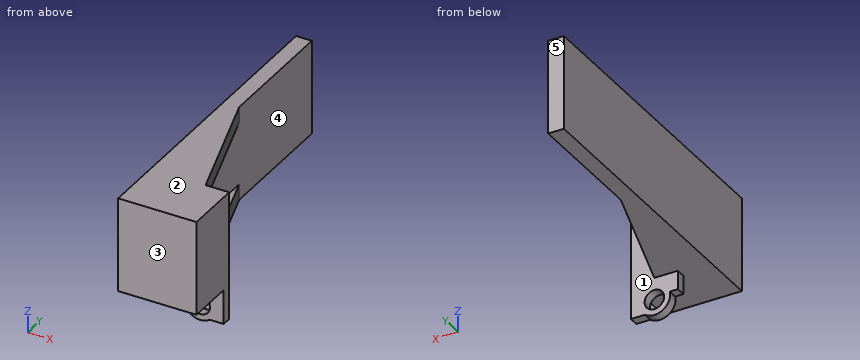
Autodesk Inventor part; units mm, degrees
ref_plane "YZ Plane" through (0, 0, 0) normal (1, 0, 0) x (0, 1, 0)
ref_plane "XZ Plane" through (0, 0, 0) normal (0, 1, 0) x (-1, 0, 0)
ref_plane "XY Plane" through (0, 0, 0) normal (0, 0, 1) x (1, 0, 0)
sketch "스케치2" plane through (0, 0, 0) normal (0, 1, 0) x (-1, 0, 0)
  circle A0 centre (0, 0) radius 3.1
  line L0 (0, 0) -> (0, 7)
  line L1 (0, 7) -> (7.475, 7)
  line L2 (7.475, 7) -> (7.475, 1.05)
  circle A1 centre (0, 0) radius 5
  line L3 (7.475, 1.05) -> (4.8885, 1.05)
  line L4 (0, 7) -> (-7.475, 7)
  line L5 (-7.475, 7) -> (-7.475, -5)
  line L6 (-7.475, -5) -> (0, -5)
  line L7 (-7.475, -5) -> (-7.475, -4)
  line L8 (-7.475, -4) -> (-3, -4)
  dimension "d0" = 6.2
  dimension "d1" = 7
  dimension "d2" = 7.475
  dimension "d3" = 5.95
  dimension "d4" = 10
  dimension "d5" = 7.475
  dimension "d21" = 1
extrude "돌출1" add sketch "스케치2" along normal blind 3 contours A1 | A1 L8 L5 L4 L0 | L0 L1 L2 L3 A1
sketch "스케치3" plane through (0, 3, 0) normal (0, 1, 0) x (1, 0, 0)
  line L0 (-7.475, -7) -> (7.475, -7)
  line L1 (-7.475, -7) -> (7.475, -7)
  line L2 (7.475, -7) -> (7.475, -37)
  line L3 (7.475, -37) -> (-7.475, -37)
  line L4 (-7.475, -37) -> (-7.475, -7)
  point P0 (0, 0)
  dimension "d8" = 30
extrude "돌출2" add sketch "스케치3" against normal blind 18
sketch "스케치11" plane through (0, 3, 0) normal (0, 1, 0) x (1, 0, 0)
  line L0 (-7.475, -37) -> (7.475, -37)
  line L1 (0, -37) -> (-17.4, -37)
  line L2 (-17.4, -37) -> (-17.4, -1.05)
  line L3 (-17.4, -1.05) -> (0, -1.05)
  line L4 (0, -1.05) -> (0, -37)
  line L5 (-7.475, -7) -> (7.475, -7)
  line L6 (-17.4, -37) -> (0, -37)
  line L7 (0, -37) -> (0, -7)
  line L8 (0, -7) -> (-17.4, -7)
  line L9 (-17.4, -7) -> (-17.4, -37)
  point P0 (0, 0)
  dimension "d40" = 17.4
extrude "돌출9" add sketch "스케치11" along normal blind 80 and the other way blind 18 contours L1 L2 L8 L5 L4 L0
sketch "스케치12" plane through (0, 83, 0) normal (0, 1, 0) x (1, 0, 0)
  line L0 (0, -7) -> (0, -37)
  line L1 (-17.4, -37) -> (0, -37)
  line L2 (0, -7) -> (-17.4, -7)
  line L3 (-17.4, -7) -> (-17.4, -37)
  line L4 (-17.4, -37) -> (0, -37)
  line L5 (0, -37) -> (0, -7)
  line L6 (-12.4, -12) -> (-5, -12)
  line L7 (-5, -12) -> (-5, -32)
  line L8 (-5, -32) -> (-12.4, -32)
  line L9 (-12.4, -32) -> (-12.4, -12)
  line L10 (-5, -12) -> (0, -12)
  line L11 (-5, -32) -> (0, -32)
  point P0 (0, 0)
  dimension "d45" = 5
extrude "돌출10" cut sketch "스케치12" against normal blind 80 contours L0 L11 L7 L10 | L7 L8 L9 L6
sketch "스케치13" plane through (7.475, -15, 37) normal (0, 0, 1) x (1, 0, 0)
  line L0 (-7.475, 18) -> (-7.475, 98)
  line L1 (-7.475, 18) -> (-19.875, 18)
  line L2 (-19.875, 18) -> (-19.875, 98)
  line L3 (-19.875, 98) -> (-19.875, 58)
  line L4 (-7.475, 18) -> (-19.875, 58)
  line L5 (-24.875, 98) -> (-7.475, 98)
  line L6 (-19.875, 98) -> (-7.475, 98)
  line L7 (-7.475, 98) -> (-7.475, 18)
  point P0 (-7.475, 15)
extrude "돌출11" cut sketch "스케치13" against normal blind 80 contours L4 L2 L5 L0
ref_plane "작업 평면5" through (7.475, -15, 52) normal (0, 0, 1) x (1, 0, 0)
sketch "스케치4" plane through (0, 3, 0) normal (0, 1, 0) x (1, 0, 0)
  line L0 (-7.475, -1.05) -> (-7.475, -37)
  line L1 (7.475, -7) -> (7.475, -37)
  line L2 (-7.475, -37) -> (7.475, -37)
  line L3 (7.475, -37) -> (7.475, -7)
  line L4 (7.475, -7) -> (-7.475, -7)
  line L5 (-7.475, -7) -> (-7.475, -37)
  line L6 (7.475, -7) -> (4.475, -7)
  line L7 (4.475, -7) -> (4.475, -37)
  line L8 (4.475, -37) -> (7.475, -37)
  line L9 (7.475, -37) -> (7.475, -7)
  point P0 (0, 0)
  dimension "d11" = 3
sketch "스케치5" plane through (-7.475, -15, 37) normal (0, 0, 1) x (1, 0, 0)
  line L0 (11.95, 18) -> (11.95, 88)
  line L1 (0, 18) -> (0, 0)
  line L2 (11.95, 53) -> (0, 18)
  point P0 (7.475, 15)
sketch "스케치6" plane through (0, -15, 0) normal (0, -1, 0) x (1, 0, 0)
  line L0 (7.475, -4) -> (3, -4)
  line L1 (7.475, 37) -> (-7.475, 37)
  line L2 (7.475, -4) -> (7, -4)
  line L3 (7, -4) -> (7, 37)
  line L4 (7, 37) -> (7.475, 37)
  line L5 (7.475, 37) -> (7.475, -4)
  dimension "d25" = 0.475
sketch "스케치7" plane through (0, 3, 0) normal (0, 1, 0) x (1, 0, 0)
  circle A0 centre (0, 0) radius 3.1
  line L0 (0, 0) -> (25, 0)
  line L1 (25, 0) -> (25, -7)
  line L2 (7, -7) -> (25, -7)
  line L3 (25, -7) -> (25, -37)
  line L4 (25, -37) -> (7, -37)
  line L5 (7, -37) -> (7, -7)
  dimension "d26" = 25
sketch "스케치8" plane through (0, 73, 0) normal (0, 1, 0) x (1, 0, 0)
  line L0 (25, -7) -> (25, -37)
  line L1 (4.475, -7) -> (4.475, -37)
  line L2 (25, -7) -> (4.475, -7)
  line L3 (4.475, -7) -> (4.475, -37)
  line L4 (4.475, -37) -> (25, -37)
  line L5 (25, -37) -> (25, -7)
  line L6 (4.475, -10) -> (-7.475, -10)
  line L7 (4.475, -10) -> (20, -10)
  line L8 (20, -10) -> (20, -34)
  line L9 (20, -34) -> (4.475, -34)
  line L10 (4.475, -34) -> (4.475, -10)
  point P0 (0, 0)
  dimension "d31" = 15.525
sketch "스케치9" plane through (4.475, 38, 37) normal (0, 0, 1) x (1, 0, 0)
  line L0 (0, 0) -> (0, 35)
  line L1 (15.525, 35) -> (15.525, -35)
  line L2 (0, 0) -> (15.525, 35)
  line L3 (15.525, 35) -> (0, 35)
  line L4 (0, 0) -> (0, 35)
  point P0 (-4.475, -38)
sketch "스케치10" plane through (-7.475, -15, 37) normal (0, 0, 1) x (1, 0, 0)
  line L0 (27.475, 88) -> (27.475, 18)
  line L1 (11.95, 53) -> (0, 18)
  line L2 (27.475, 88) -> (0, 18)
  line L3 (0, 18) -> (27.475, 18)
  line L4 (32.475, 88) -> (27.475, 88)
  line L5 (27.475, 18) -> (27.475, 88)
  line L6 (27.475, 88) -> (27.475, 53)
  line L7 (0, 18) -> (27.475, 53)
  line L8 (0, 18) -> (11.95, 53)
  line L9 (27.475, 88) -> (11.95, 53)
  point P0 (7.475, 15)
ref_plane "작업 평면4" through (7.475, 3, 82) normal (0, 0, -1) x (-1, 0, 0)
properties part number "motor_limit_1"
Check sheet for the modelled part. Datum: model origin and axes. Units: mm. Face numbers are marked on the shaded views. A direction names the side the tool comes from. Round coordinates to 2 decimals unless told otherwise and drop trailing zeros. Loops run counter-clockwise (first coordinate to the right, second up) from the corner with the lowest first, then second, coordinate; pieces in that order, holes last. Notation, with made-up numbers: M 47.25,23.25 L 86.25,23.25 A12 cw 86.25,36.25 Z; hole C -40,48.5 d6. An arc over 180 degrees is marked long. Answer as a JSON object with one key per item and string values.
1. Section check A-A (z = 0). Record the boundary of the cut face in (x, y) (3 decimals).
Reply:
{"outline": "M -5,0 L -3.1,0 L -3.1,3 L -5,3 Z; M 3.1,0 L 7.475,0 L 7.475,3 L 3.1,3 Z"}
2. Section check C-C (x = 6). Record the boundary of the cut face in (y, z), plus the area to 3 significant figures.
Reply:
{"outline": "M -15,7 L 0,7 L 0,-4 L 3,-4 L 3,37 L -15,37 Z", "area": "573 mm²"}
3. Access from +Z, -Z, +X, -X, +Y, -Y to the whole of each face (thin tool, end or side, straight path). Record for the marked faces 4 and 5.
Reply:
{"face 4": "+X, +Y", "face 5": "+Z, -Z, +X, -X, +Y"}
4. Scan lines: line 1 (Z direction, x = 0, y = 0.6); line 2 (X direction, y = 1.6, z = 0) (3 decimals); line 3 (Y direction, x = -4.25, z = 12.5). Record each from-to range of solid material in increasing order.
Reply:
{"line 1": "z = -5 to -3.1, 3.1 to 37", "line 2": "x = -5 to -3.1, 3.1 to 7.475", "line 3": "y = -15 to 3"}
5. Section check D-D (z = 9.5). Record the boundary of the cut face in (x, y) (3 decimals), plus the area to 3 significant figures.
Reply:
{"outline": "M -17.4,-15 L 7.475,-15 L 7.475,3 L 0,3 L -12.4,43 L -12.4,83 L -17.4,83 Z", "area": "1,100 mm²"}
6. Gauge pin test, flat ends, axial feed: P1, Ø9.5, axis at x = 2, z = -1.5, coming from the -Y side; P2, Ø1.5, axis at x = 4.5, y = 1.5, coming from the -Z side; P3, Ø1.3, axis at x = -6.5, y = 2, coming from the -Z side; P4, Ø10, axis at y = 49.5, z = 2.5, coming from the -X side. Record the tip position at first contact, or that the pin passes through.
Reply:
{"P1": "stops at y = 0", "P2": "stops at z = -4", "P3": "stops at z = 1.05", "P4": "stops at x = -17.4"}
7. Mould release check, pull along Z, two halves, no side actions. Record for the marked faces 1, 2 and 3: pulls with the +Z half, pulls with the -Z half, needs draft (parallel to the pull), parting line crosses it, or undercut.
Reply:
{"face 1": "undercut", "face 2": "pulls with the +Z half", "face 3": "needs draft"}
8. Section check B-B (y = 36). Record the boundary of the cut face in (x, z).
Reply:
{"outline": "M -17.4,7 L -10.23,7 L -10.23,12 L -12.4,12 L -12.4,32 L -10.23,32 L -10.23,37 L -17.4,37 Z"}
